Autodesk Inventor part; units mm, degrees
ref_plane "YZ Plane" through (0, 0, 0) normal (1, 0, 0) x (0, 1, 0)
ref_plane "XZ Plane" through (0, 0, 0) normal (0, 1, 0) x (-1, 0, 0)
ref_plane "XY Plane" through (0, 0, 0) normal (0, 0, 1) x (1, 0, 0)
sketch "Sketch1" plane through (0, 0, 0) normal (0, 0, 1) x (1, 0, 0)
  circle A0 centre (300, 45) radius 3
  circle A1 centre (-300, -45) radius 3
  circle A2 centre (300, -45) radius 3
  circle A3 centre (-300, 45) radius 3
  line L0 (395, -87) -> (-395, -87)
  line L1 (395, -87) -> (395, 87)
  line L2 (-395, 87) -> (395, 87)
  line L3 (-395, 87) -> (-395, -87)
  line L4 (395, 87) -> (-395, 87)
  line L5 (-395, 87) -> (-395, -148)
  line L6 (-395, -148) -> (395, -148)
  line L7 (395, -148) -> (395, 87)
  point P0 (0, 0)
  dimension "d0" = 235
extrude "Extrusion1" add sketch "Sketch1" along normal blind 8
sketch "Sketch2" plane through (0, 0, 8) normal (0, 0, 1) x (1, 0, 0)
  line L0 (387.8577, -133.54) -> (-386.877, -133.54) construction
  line L1 (390.6938, 247.5) -> (-382.1387, 247.5) construction
  arc A0 (355.5754, 239.7531) -> (355.5754, 255.2469) centre (355.5754, 247.5) ccw
  arc A1 (304.8389, 255.2469) -> (304.8389, 239.7531) centre (304.8389, 247.5) ccw
  line L2 (355.5754, 239.7531) -> (304.8389, 239.7531)
  line L3 (304.8389, 255.2469) -> (355.5754, 255.2469)
  line L4 (-310.6878, 239.7531) -> (-360.707, 239.7531)
  line L5 (-360.707, 255.2469) -> (-310.6878, 255.2469)
  arc A2 (-310.6878, 239.7531) -> (-310.6878, 255.2469) centre (-310.6878, 247.5) ccw
  arc A3 (-360.707, 255.2469) -> (-360.707, 239.7531) centre (-360.707, 247.5) ccw
  line L6 (304.8389, -133.54) -> (355.5754, -133.54) construction
  line L7 (304.8389, -141.2869) -> (355.5754, -141.2869)
  line L8 (355.5754, -125.7931) -> (304.8389, -125.7931)
  arc A4 (304.8389, -125.7931) -> (304.8389, -141.2869) centre (304.8389, -133.54) ccw
  arc A5 (355.5754, -141.2869) -> (355.5754, -125.7931) centre (355.5754, -133.54) ccw
  line L9 (-360.707, -133.54) -> (-310.6878, -133.54) construction
  line L10 (-360.707, -141.2869) -> (-310.6878, -141.2869)
  line L11 (-310.6878, -125.7931) -> (-360.707, -125.7931)
  arc A6 (-360.707, -125.7931) -> (-360.707, -141.2869) centre (-360.707, -133.54) ccw
  arc A7 (-310.6878, -141.2869) -> (-310.6878, -125.7931) centre (-310.6878, -133.54) ccw
  point P0 (0, 0)
  point P1 (330.2072, -133.54)
  point P2 (-335.6974, -133.54)
  dimension "d3" = 381.04
extrude "Extrusion2" cut sketch "Sketch2" against normal through all contours A4 L8 A5 L7 | A6 L11 A7 L10
thicken "Thicken1" operation add thickness 4 both sides no extend neighbours no toward (0, -1, 0) faces at (-131.6667, -148, 2.6667)
fillet "Fillet1" radius 2 4 edges at (395, -152, 4) (395, 87, 4) (-395, -152, 4) (-395, 87, 4)
properties part number "Plexi_Bildverarbeitungsband"
Can you work these out from the model? Positions are in its coordinate system, mm. Round coordinates to 2 decimals unless told otherwise and drop trailing zeros. Loops run counter-clockwise (first coordinate to the right, second up) from the corner with the lowest first, then second, coordinate; pieces in that order, holes last. Notation, with made-up numbers: M 89,-16 L 126,-16 A9 cw 126,-8 Z; hole C -37,69.25 d10. An arc over 180 degrees is marked long. Write item = value, one per line. Start each with the question number.
(1) Suppose I cut it at A-A on x = -323. Write out the boundary of the cut face in (y, z), plus the area to 3 significant figures.
(2) I'm going to push a flat-ended pin straight in: P1, Ø1.5, axis at x = 196, y = 33, coming from the -Z side. Where does the tip first touch, or does it pass through?
(3) Suppose I cut it at B-B on y = -133.54. Write out the boundary of the cut face in (x, z), plus the area to 3 significant figures.
(4) I need wall thicknesses on line 1 along Y through (x, z) = (-300, 3); line 2 along Y through (x, z) = (315, 5.25); line 3 along Y through (x, z) = (300, 1.5). Which ranges of each line are inside material? Lowest first, please.
Answer block:
q1.outline = M -152,0 L -141.29,0 L -141.29,8 L -152,8 Z; M -125.79,0 L 87,0 L 87,8 L -125.79,8 Z
q1.area = 1,790 mm²
q2.P1 = 0
q3.outline = M -395,0 L -368.45,0 L -368.45,8 L -395,8 Z; M -302.94,0 L 297.09,0 L 297.09,8 L -302.94,8 Z; M 363.32,0 L 395,0 L 395,8 L 363.32,8 Z
q3.area = 5,270 mm²
q4.line_1 = -152 to -48, -42 to 42, 48 to 87
q4.line_2 = -152 to -141.29, -125.79 to 87
q4.line_3 = -152 to -139.59, -127.49 to -48, -42 to 42, 48 to 87
